```python
from build123d import *

# Parameters (mm, degrees)
EXTRUDE1_DEPTH     = 0.9
EXTRUDE2_DEPTH     = 0.9
SKETCH3_R          = 1.346200001
CUT_EXTRUDE2_DEPTH = 1.9
EXTRUDE3_DEPTH     = 1.9
CUT_EXTRUDE3_DEPTH = 1.9
FILLET1_R          = 0.5
CUT_EXTRUDE4_DEPTH = 1.9


with BuildPart() as part:
    # Sketch1 → Extrude1 (new body)
    with BuildSketch(Plane.XY):
        Polygon((-16.337044405, 167.45476352), (16.337044405, 167.45476352), (16.002062475, 162.343926895), (-16.002062475, 162.343926895), align=None)
    extrude(amount=EXTRUDE1_DEPTH)

    # Sketch2 → Extrude2 (add)
    with BuildSketch(Plane(origin=(0, 0, 0), x_dir=(-1, 0, 0), z_dir=(0, 0, -1))):
        with BuildLine():
            Line((16.84417657, 175.192105175), (15.717346464, 158))
            Line((15.717346464, 158), (-15.717346464, 158))
            Line((-15.717346464, 158), (-16.84417657, 175.192105175))
            ThreePointArc((-16.84417657, 175.192105175), (0, 176), (16.84417657, 175.192105175))
        make_face()
    extrude(amount=-EXTRUDE2_DEPTH)

    # Sketch3 → Cut-Extrude2 (cut, through all)
    with BuildSketch(Plane.XY):
        with Locations((-2.271044833, 173.485135834)):
            Circle(SKETCH3_R)
        with BuildLine():
            Line((-1.704039652, 160.491487345), (-1.690948935, 159.491487345))
            ThreePointArc((-1.690948935, 159.491487345), (-2.082595001, 159.089451413), (-2.484630933, 159.481097479))
            Line((-2.484630933, 159.481097479), (-2.49772165, 160.481097479))
            ThreePointArc((-2.49772165, 160.481097479), (-2.106075584, 160.883133411), (-1.704039652, 160.491487345))
        make_face()
    extrude(amount=CUT_EXTRUDE2_DEPTH, mode=Mode.SUBTRACT)

    # Sketch4 → Extrude3 (cut, through all)
    with BuildSketch(Plane.XY.offset(0.9)):
        with BuildLine():
            Line((-12, 175.590432541), (-12, 171))
            ThreePointArc((-12, 171), (-12.292893219, 170.292893219), (-13, 170))
            Line((-13, 170), (-16.503868017, 170))
            Line((-16.503868017, 170), (-16.84417657, 175.192105175))
            ThreePointArc((-16.84417657, 175.192105175), (-14.423463408, 175.407992131), (-12, 175.590432541))
        make_face()
    extrude(amount=-EXTRUDE3_DEPTH, mode=Mode.SUBTRACT)

    # Sketch5 → Cut-Extrude3 (cut, through all)
    with BuildSketch(Plane.XY.offset(0.9)):
        with BuildLine():
            Line((-5.934879033, 175.899906796), (-5.934879033, 173.754533822))
            Line((-5.934879033, 173.754533822), (-13.425811407, 173.754533822))
            Line((-13.425811407, 173.754533822), (-13.425811407, 175.487172147))
            ThreePointArc((-13.425811407, 175.487172147), (-9.682544658, 175.733458194), (-5.934879033, 175.899906796))
        make_face()
    extrude(amount=-CUT_EXTRUDE3_DEPTH, mode=Mode.SUBTRACT)

    # Fillet1
    fillet1_edges = [part.edges().sort_by_distance(p)[0] for p in [
        (-5.934879033, 173.754533822, 0.45),
    ]]
    fillet(fillet1_edges, radius=FILLET1_R)

    # Sketch6 → Cut-Extrude4 (cut, through all)
    with BuildSketch(Plane(origin=(0, 0, 0), x_dir=(-1, 0, 0), z_dir=(0, 0, -1))):
        with BuildLine():
            Line((3.939992499, 158), (4.387488465, 175.945303845))
            ThreePointArc((4.387488465, 175.945303845), (5.161233662, 175.924306641), (5.934879033, 175.899906796))
            Line((5.934879033, 175.899906796), (5.934879033, 174.254533822))
            ThreePointArc((5.934879033, 174.254533822), (6.081325642, 173.900980431), (6.434879033, 173.754533822))
            Line((6.434879033, 173.754533822), (12, 173.754533822))
            Line((12, 173.754533822), (12, 171))
            ThreePointArc((12, 171), (12.292893219, 170.292893219), (13, 170))
            Line((13, 170), (16.503868017, 170))
            Line((16.503868017, 170), (15.717346464, 158))
            Line((15.717346464, 158), (3.939992499, 158))
        make_face()
    extrude(amount=-CUT_EXTRUDE4_DEPTH, mode=Mode.SUBTRACT)


solid = part.part
```
Work out the finished part from the listing and answer in its coordinate system (mm). A direction names the side the tool comes from. Round coordinates to 2 decimals unless told otherwise and drop trailing zeros. Loops run counter-clockwise (first coordinate to the right, second up) from the corner with the lowest first, then second, coordinate; pieces in that order, holes last.
(1) Find the intervals of material crossed by L1, parallel to Y at x = -2.25, z = 0.6; L2, parallel to X at y = 160.75, z = 0.15; L3, parallel to X at y = 173.5, z = 0.55, in increasing order.
Computed values:
L1: y = 158 to 159.12, 160.85 to 172.14, 174.83 to 175.99
L2: x = -4.01 to -2.4, -1.8 to 15.9
L3: x = -4.33 to -3.62, -0.92 to 16.73
(2) The mould has two halves that part along X. Classify faces 3 (the flat face through (6, 167, 0)), 4 (the cylindrical face through (-2.56, 172.17, 0.44)): pulls with the +X half, pulls with the -X half, needs draft (parallel to the pull), parting line crosses it, or undercut.
Computed values:
face 3: needs draft
face 4: undercut
(3) The part is cut by section D-D, the plane y = 169. Give the vertices of the cut face in (x, z).
Computed values:
outline: (-4.21, 0) - (16.44, 0) - (16.44, 0.9) - (-4.21, 0.9) - close
(4) Each of these flat-tipped pins is pushed along its axis until it touches: P1, Ø2.5, axis at x = -2.27, y = 173.49, coming from the +Z side; P2, Ø1, axis at x = 6.5, y = 165, coming from the -Z side. Where does it stop, or does it pass through?
Computed values:
P1: passes through
P2: stops at z = 0
(5) The part is cut by section A-A, the plane x = -2.25. Give the vertices of the cut face in (y, z), and give its area (3 significant figures).
Computed values:
outline: (158, 0) - (159.12, 0) - (159.12, 0.9) - (158, 0.9) - close; (160.85, 0) - (172.14, 0) - (172.14, 0.9) - (160.85, 0.9) - close; (174.83, 0) - (175.99, 0) - (175.99, 0.9) - (174.83, 0.9) - close
area: 12.2 mm2
(6) The part is cut by section C-C, the plane y = 174.5. Give the vertices of the cut face in (x, z), and give its area (3 significant figures).
Computed values:
outline: (-4.35, 0) - (-3.16, 0) - (-3.16, 0.9) - (-4.35, 0.9) - close; (-1.39, 0) - (16.8, 0) - (16.8, 0.9) - (-1.39, 0.9) - close
area: 17.4 mm2
(7) The part is cut by section B-B, the plane z = 0.75. Give the vertices of the cut face in (x, y), and give its area (3 significant figures).
Computed values:
outline: (-4.39, 175.95) - (-3.94, 158) - (15.72, 158) - (16.84, 175.19) arc R176 ccw to start; hole circle Ø2.69 at (-2.27, 173.49); hole (-2.5, 160.48) - (-2.48, 159.48) arc R0.4 ccw to (-1.69, 159.49) - (-1.7, 160.49) arc R0.4 ccw to start
area: 357 mm2
(8) For faces 1 (the flat face through (5.8, 158, 0.4)), 2 (the cylindrical face through (6.388, 175.884, 0.444)), determine the directions among +Z, -Z, +X, -X, +Y, -Y from which every point of the face is accessible in a straight line to the end or side of a thin tool.
Computed values:
face 1: +Z, -Z, +X, -X, -Y
face 2: +Z, -Z, +Y
